Geometry: final body of the model. Coordinates: model frame, mm. A direction names the side the tool comes from. Coordinates: 2 decimals unless noted, no trailing zeros. Order: outer loops, then holes, each group sorted by start corner. A loop starts at its lowest first (then second) coordinate and runs counter-clockwise, first axis right, second up. Notation, with made-up numbers: M 32.25,-6.5 L 71.25,-6.5 A34 ccw 71.25,27.5 Z; hole C 29,14 d3. An arc over 180 degrees is marked long. Write item = value, one per line.
from build123d import *

# Parameters (mm, degrees)
F0_W      = 100
F0_H      = 150
F1_DEPTH  = 5
F2_R      = 1.5
F3_DEPTH  = 25
F4_R      = 2.5
F4_R_2    = 1.5
F5_DEPTH  = 3
F6_R      = 2.75
F7_DEPTH  = 2.5
F8_W      = 3
F8_H      = 10
F8_W_2    = 5
F8_H_2    = 3
F8_W_3    = 10
F9_DEPTH  = 25
F10_W     = 55.5
F10_H     = 137
F10_W_2   = 53.5
F10_H_2   = 135
F11_DEPTH = 1
F12_W     = 1
F12_H     = 6
F13_DEPTH = 5
F14_DEPTH = 12.5
F15_R     = 4
F16_DEPTH = 25
F17_W     = 9.35
F17_H     = 6
F18_DEPTH = 2
F19_W     = 5
F19_H     = 10
F20_DEPTH = 12
F21_R     = 1.5
F22_DEPTH = 150
F24_DEPTH = 2.5
F26_DEPTH = 2.5
F28_DEPTH = 150
F29_R     = 1.5
F30_DEPTH = 25
F31_R     = 3
F32_DEPTH = 2.5


# Not quite as in the source:
# - a feature names something its author has since deleted; it is built from what else it names


with BuildPart() as f1:
    # F0 (on Top) → F1 (new body)
    with BuildSketch(Plane.XY):
        Rectangle(F0_W, F0_H)
    extrude(amount=F1_DEPTH)

    # F2 (on face) → F3 (cut)
    with BuildSketch(Plane.XY.offset(5)):
        with Locations((-32, 56.5)):
            Circle(F2_R)
        with Locations((7.5, 56.5)):
            Circle(F2_R)
        with Locations((-32, -58.5)):
            Circle(F2_R)
        with Locations((7.5, -58.5)):
            Circle(F2_R)
    extrude(amount=-F3_DEPTH, mode=Mode.SUBTRACT)

    # F4 (on face) → F5 (join)
    with BuildSketch(Plane.XY.offset(5)):
        with Locations((-32, -58.5)):
            Circle(F4_R)
        with Locations((-32, -58.5)):
            Circle(F4_R_2, mode=Mode.SUBTRACT)
        with Locations((7.5, -58.5)):
            Circle(F4_R)
        with Locations((7.5, -58.5)):
            Circle(F4_R_2, mode=Mode.SUBTRACT)
        with Locations((7.5, 56.5)):
            Circle(F4_R)
        with Locations((7.5, 56.5)):
            Circle(F4_R_2, mode=Mode.SUBTRACT)
        with Locations((-32, 56.5)):
            Circle(F4_R)
        with Locations((-32, 56.5)):
            Circle(F4_R_2, mode=Mode.SUBTRACT)
    extrude(amount=F5_DEPTH)

    # F6 (on face) → F7 (cut)
    with BuildSketch(Plane(origin=(0, 0, 0), x_dir=(1, 0, 0), z_dir=(0, 0, -1))):
        with Locations((-32, 58.5)):
            Circle(F6_R)
        with Locations((7.5, 58.5)):
            Circle(F6_R)
        with Locations((-32, -56.5)):
            Circle(F6_R)
        with Locations((7.5, -56.5)):
            Circle(F6_R)
    extrude(amount=-F7_DEPTH, mode=Mode.SUBTRACT)

    # F8 (on face) → F9 (cut)
    with BuildSketch(Plane.XY.offset(5)):
        with Locations((-46.5, 62.5)):
            Rectangle(F8_W, F8_H)
        with Locations((-46.5, 27.5)):
            Rectangle(F8_W, F8_H)
        with Locations((-46.5, -27.5)):
            Rectangle(F8_W, F8_H)
        with Locations((-46.5, -62.5)):
            Rectangle(F8_W, F8_H)
        with Locations((2.5, 71.5)):
            Rectangle(F8_W_2, F8_H_2)
        with Locations((-2.5, 71.5)):
            Rectangle(F8_W_2, F8_H_2)
        with Locations((2.5, -71.5)):
            Rectangle(F8_W_2, F8_H_2)
        with Locations((-2.5, -71.5)):
            Rectangle(F8_W_2, F8_H_2)
        with Locations((46.5, 62.5)):
            Rectangle(F8_W, F8_H)
        with Locations((46.5, -62.5)):
            Rectangle(F8_W, F8_H)
        with Locations((46.5, -27.5)):
            Rectangle(F8_W, F8_H)
        with Locations((46.5, 27.5)):
            Rectangle(F8_W, F8_H)
        with Locations((-30, 71.5)):
            Rectangle(F8_W_3, F8_H_2)
        with Locations((30, 71.5)):
            Rectangle(F8_W_3, F8_H_2)
        with Locations((30, -71.5)):
            Rectangle(F8_W_3, F8_H_2)
        with Locations((-30, -71.5)):
            Rectangle(F8_W_3, F8_H_2)
    extrude(amount=-F9_DEPTH, mode=Mode.SUBTRACT)

    # F10 (on face) → F11 (join)
    with BuildSketch(Plane.XY.offset(5)):
        with Locations((-12.25, -1)):
            Rectangle(F10_W, F10_H)
        with Locations((-12.25, -1)):
            Rectangle(F10_W_2, F10_H_2, mode=Mode.SUBTRACT)
    extrude(amount=F11_DEPTH)

    # F12 (on face) → F13 (join)
    with BuildSketch(Plane.XY.offset(5)):
        Polygon((34.85, 45), (25.5, 45), (25.5, 43), (26.5, 43), (26.5, 37), (25.5, 37), (25.5, 35), (34.85, 35), (34.85, 37), (33.85, 37), (33.85, 43), (34.85, 43), align=None)
        with Locations((26, 40)):
            Rectangle(F12_W, F12_H)
        with Locations((34.35, 40)):
            Rectangle(F12_W, F12_H)
    extrude(amount=F13_DEPTH)

    # F12 (on face) → F14 (cut, symmetric)
    with BuildSketch(Plane.XY.offset(5)):
        with Locations((34.35, 40)):
            Rectangle(F12_W, F12_H)
        with Locations((26, 40)):
            Rectangle(F12_W, F12_H)
    extrude(amount=F14_DEPTH, both=True, mode=Mode.SUBTRACT)

    # F15 (on face) → F16 (cut)
    with BuildSketch(Plane.XZ.offset(-35)):
        with Locations((30.175, 10)):
            Circle(F15_R)
    extrude(amount=-F16_DEPTH, mode=Mode.SUBTRACT)

    # F17 (on face) → F18 (cut)
    with BuildSketch(Plane(origin=(0, 0, 0), x_dir=(1, 0, 0), z_dir=(0, 0, -1))):
        with Locations((30.175, -40)):
            Rectangle(F17_W, F17_H)
    extrude(amount=-F18_DEPTH, mode=Mode.SUBTRACT)

    # F19 (on face) → F20 (join)
    with BuildSketch(Plane.XY.offset(5)):
        with Locations((42.4, 60)):
            Rectangle(F19_W, F19_H)
        with Locations((-42.4, 60)):
            Rectangle(F19_W, F19_H)
        with Locations((-42.4, -60)):
            Rectangle(F19_W, F19_H)
        with Locations((42.4, -60)):
            Rectangle(F19_W, F19_H)
    extrude(amount=F20_DEPTH)

    # F21 (on face) → F22 (cut)
    with BuildSketch(Plane.YZ.offset(44.9)):
        with Locations((-60, 10)):
            Circle(F21_R)
        with Locations((60, 10)):
            Circle(F21_R)
    extrude(amount=-F22_DEPTH, mode=Mode.SUBTRACT)

    # F23 (on face) → F24 (cut)
    with BuildSketch(Plane(origin=(39.9, 0, 0), x_dir=(0, -1, 0), z_dir=(-1, 0, 0))):
        Polygon((-58.4122867597, 12.75), (-61.5877132403, 12.75), (-63.1754264805, 10), (-61.5877132403, 7.25), (-58.4122867597, 7.25), (-56.8245735195, 10), align=None)
        Polygon((61.5877132403, 7.25), (63.1754264805, 10), (61.5877132403, 12.75), (58.4122867597, 12.75), (56.8245735195, 10), (58.4122867597, 7.25), align=None)
    extrude(amount=-F24_DEPTH, mode=Mode.SUBTRACT)

    # F25 (on face) → F26 (cut)
    with BuildSketch(Plane.YZ.offset(-39.9)):
        Polygon((-58.4122867597, 12.75), (-61.5877132403, 12.75), (-63.1754264805, 10), (-61.5877132403, 7.25), (-58.4122867597, 7.25), (-56.8245735195, 10), align=None)
        Polygon((61.5877132403, 7.25), (63.1754264805, 10), (61.5877132403, 12.75), (58.4122867597, 12.75), (56.8245735195, 10), (58.4122867597, 7.25), align=None)
    extrude(amount=-F26_DEPTH, mode=Mode.SUBTRACT)

    # F27 (on face) → F28 (cut)
    with BuildSketch(Plane.YZ.offset(44.9)):
        with BuildLine():
            ThreePointArc((-65, 10), (-60, 15), (-55, 10))
            Line((-55, 10), (-55, 17))
            Line((-55, 17), (-65, 17))
            Line((-65, 17), (-65, 10))
        make_face()
        with BuildLine():
            ThreePointArc((55, 10), (60, 15), (65, 10))
            Line((65, 10), (65, 17))
            Line((65, 17), (55, 17))
            Line((55, 17), (55, 10))
        make_face()
    extrude(amount=-F28_DEPTH, mode=Mode.SUBTRACT)

    # F29 (on face) → F30 (cut)
    with BuildSketch(Plane.XY.offset(5)):
        with Locations((-35, 62.5)):
            Circle(F29_R)
        with Locations((35, 62.5)):
            Circle(F29_R)
        with Locations((-35, -64.5)):
            Circle(F29_R)
        with Locations((35, -64.5)):
            Circle(F29_R)
    extrude(amount=-F30_DEPTH, mode=Mode.SUBTRACT)

    # F31 (on face) → F32 (cut)
    with BuildSketch(Plane.XY.offset(5)):
        with Locations((35, -64.5)):
            Circle(F31_R)
        with Locations((35, 62.5)):
            Circle(F31_R)
        with Locations((-35, 62.5)):
            Circle(F31_R)
        with Locations((-35, -64.5)):
            Circle(F31_R)
    extrude(amount=-F32_DEPTH, mode=Mode.SUBTRACT)


solid = f1.part
1) Section C-C, the plane x = -12. Return loops of the section in (y, z), and give its area (3 significant figures).
Numbers:
outline = M -75,0 L 75,0 L 75,5 L 67.5,5 L 67.5,6 L 66.5,6 L 66.5,5 L -68.5,5 L -68.5,6 L -69.5,6 L -69.5,5 L -75,5 Z
area = 752 mm²
2) Mould query, pull axis Y, two halves, no side actions, for faces 1 (the face through (-39.9, 57.7, 12.4)), 2 (the face through (-45, 62, 3)). Classes: pulls with the +Y half, pulls with the -Y half, needs draft (parallel to the pull), parting line crosses it, or undercut.
Numbers:
face_1 = needs draft
face_2 = undercut
3) Section A-A, the plane x = 7.5. Give the number of separate pieces and of enclosed holes in the cut face, and give its area (4 significant figures).
Numbers:
separate_pieces = 3
enclosed_holes = 0
area = 721.5 mm²
4) Pin query (flat end, axial travel): pin 1 (0.5 mm diameter, centred on y = 31, z = 5.5, fed in from -X); pin 2 (8 mm diameter, centred on x = -3, y = -7, fed in from +Z); pin 3 (5 mm diameter, centred on y = -60, z = 10, fed in from -X). Return the tip coordinate at first contact, or that it passes through.
Numbers:
pin_1 = -40
pin_2 = 5
pin_3 = -44.9
5) Line query: L1, parallel to Z at x = -43, y = 60; L2, parallel to Y at x = -29, z = 4.75; L3, parallel to X at y = 55.5, z = 10.5. Output: solid intervals per line, ascending.
Numbers:
L1 = 0 to 8.5, 11.5 to 15
L2 = -75 to -73, -70 to 70, 73 to 75
L3 = -44.9 to -39.9, 39.9 to 44.9
6) Set-up query: faces 3 (the face through (7.142, 53.773, 1.232)), 4 (the face through (42, 55, 7)), 5 (the face through (-48, 27, 3)). Return all of +Z, -Z, +X, -X, +Y, -Y with unobstructed straight access to the full face (end or side cutting, diameter ignored); none if empty.
Numbers:
face_3 = -Z
face_4 = +Z, +X
face_5 = +Z, -Z
7) Section B-B, the plane y = -12. Return loops of the section in (x, z).
Numbers:
outline = M -50,0 L 50,0 L 50,5 L 15.5,5 L 15.5,6 L 14.5,6 L 14.5,5 L -39,5 L -39,6 L -40,6 L -40,5 L -50,5 Z
